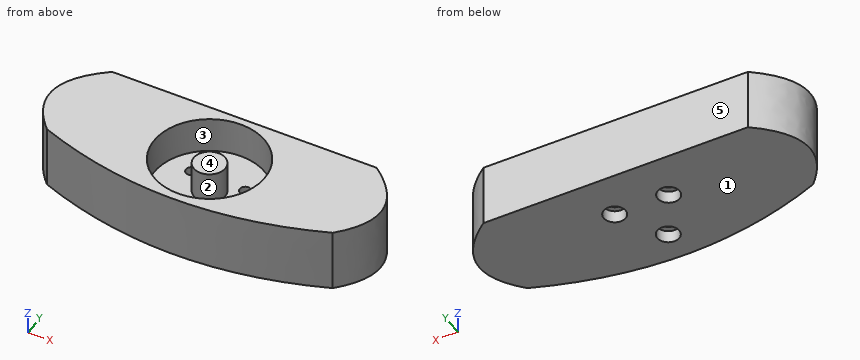
from build123d import *

# Parameters (mm, degrees)
BOSS_EXTRUDE1_DEPTH                              = 20
SKETCH4_R                                        = 17.5
CUT_EXTRUDE1_DEPTH                               = 11.453250926
SKETCH5_R                                        = 5
BOSS_EXTRUDE2_DEPTH                              = 10
CBORE_FOR_M5_HEX_HEAD_MACHINE_SCREW2_D           = 3.5
CBORE_FOR_M5_HEX_HEAD_MACHINE_SCREW2_DEPTH       = 11
CBORE_FOR_M5_HEX_HEAD_MACHINE_SCREW2_CBORE_D     = 7
CBORE_FOR_M5_HEX_HEAD_MACHINE_SCREW2_CBORE_DEPTH = 4
CBORE_FOR_M5_HEX_HEAD_MACHINE_SCREW2_TIP         = 1.75


with BuildPart() as part:
    # Sketch2 → Boss-Extrude1 (new body)
    with BuildSketch(Plane.XY):
        with BuildLine():
            Line((42.376776125, 8.683218748), (-42.540089832, 8.683218747))
            add(Edge.make_bspline(
                [(-42.540089832, 8.683218747), (-61.647606257, -6.072667773), (-45.873698376, -22.15549797)],
                knots=[0, 0, 0, 1, 1, 1], degree=2))
            add(Edge.make_bspline(
                [(-45.873698376, -22.15549797), (0.203235462, -40.398996626), (45.873698397, -22.155497949)],
                knots=[0, 0, 0, 1, 1, 1], degree=2))
            add(Edge.make_bspline(
                [(45.873698397, -22.155497949), (61.713202875, -6.005950809), (42.376776125, 8.683218748)],
                knots=[0, 0, 0, 1, 1, 1], degree=2))
        make_face()
    extrude(amount=BOSS_EXTRUDE1_DEPTH)

    # Sketch4 → Cut-Extrude1 (cut)
    with BuildSketch(Plane.XY.offset(20)):
        with Locations((0, -11.063024907)):
            Circle(SKETCH4_R)
    extrude(amount=-CUT_EXTRUDE1_DEPTH, mode=Mode.SUBTRACT)

    # Sketch5 → Boss-Extrude2 (add)
    with BuildSketch(Plane.XY.offset(8.546749074)):
        with Locations((0, -11.063024907)):
            Circle(SKETCH5_R)
    extrude(amount=BOSS_EXTRUDE2_DEPTH)

    # CBORE for M5 Hex Head Machine Screw2
    with Locations(Plane(origin=(0, 0, 0), x_dir=(-1, 0, 0), z_dir=(0, 0, -1))):
        with Locations((-8.660254038, -6.129479586), (0, -21.129479586), (8.660254038, -6.129479586)):
            CounterBoreHole(CBORE_FOR_M5_HEX_HEAD_MACHINE_SCREW2_D / 2, CBORE_FOR_M5_HEX_HEAD_MACHINE_SCREW2_CBORE_D / 2, CBORE_FOR_M5_HEX_HEAD_MACHINE_SCREW2_CBORE_DEPTH, depth=CBORE_FOR_M5_HEX_HEAD_MACHINE_SCREW2_DEPTH)
            with Locations((0, 0, -(CBORE_FOR_M5_HEX_HEAD_MACHINE_SCREW2_DEPTH + CBORE_FOR_M5_HEX_HEAD_MACHINE_SCREW2_TIP / 2))):  # 90° drill point
                Cone(0, CBORE_FOR_M5_HEX_HEAD_MACHINE_SCREW2_D / 2, CBORE_FOR_M5_HEX_HEAD_MACHINE_SCREW2_TIP, mode=Mode.SUBTRACT)


solid = part.part
Geometry: final body of the model. Coordinates: model frame, mm. Face numbers are marked on the shaded views. A direction names the side the tool comes from. Round coordinates to 2 decimals unless told otherwise and drop trailing zeros. Put each result on its own line as item: value. Start each with the question number.
Q1. Reachability of the marked faces 1 and 2 from +Z, -Z, +X, -X, +Y, -Y: full face, straight path, thin tool, end or side. Return the list, or none.
Q2. First-contact query: pin 1 (4 mm diameter, centred on x = -8.66, y = -6.13, fed in from -Z); pin 2 (1 mm diameter, centred on y = -2.5, z = 8.5, fed in from -X); pin 3 (4.5 mm diameter, centred on x = 0, y = -21.13, fed in from +Z). Flat tips, straight axial feed; report the tip coordinate or a pass-through.
Q3. Section A-A on z = 2.5. Give the number of separate pieces and of enclosed holes in the cut face, and give its area (3 significant figures).
Q4. Line query: probe 1 along X at (y, z) = (-9.5, 16); probe 2 along X at (y, z) = (-12.5, 12); probe 3 along Z at (x, y) = (5, -19.5). Output: solid intervals per line, ascending.
Q5. Pull-direction query (X, two-part tool) for the marked faces 3, 4 and 5; classes: +X half, -X half, draft (parallel to the pull), parting line (faces both ways), or undercut.
Ans:
1. face 1: -Z, +X, -X, +Y, -Y
1. face 2: +Z
2. pin 1: stops at z = 4
2. pin 2: stops at x = -52.13
2. pin 3: stops at z = 8.55
3. separate pieces: 1
3. enclosed holes: 3
3. area: 3,530 mm2
4. probe 1: x = -52.91 to -17.43, -4.75 to 4.75, 17.43 to 52.91
4. probe 2: x = -52.24 to -17.44, -4.79 to 4.79, 17.44 to 52.24
4. probe 3: z = 0 to 8.55
5. face 3: undercut
5. face 4: undercut
5. face 5: draft
